Work out the finished part from the listing and answer in its coordinate system (mm). A direction names the side the tool comes from. Round coordinates to 2 decimals unless told otherwise and drop trailing zeros. Loops run counter-clockwise (first coordinate to the right, second up) from the corner with the lowest first, then second, coordinate; pieces in that order, holes last. Notation, with made-up numbers: (81.5, 39.5) -> (119.5, 39.5) arc R22 cw to (119.5, 51.5) -> close; hole circle Ø8 at (50.25, -35). An arc over 180 degrees is marked (long way). Use one line per item in the form item = value.
```python
from build123d import *

# Parameters (mm, degrees)
F0_W      = 60
F0_H      = 30
F0_W_2    = 30
F0_H_2    = 60
F1_DEPTH  = 20
F3_DEPTH  = 5
F4_W      = 5
F4_H      = 5
F5_DEPTH  = 15
F6_W      = 5
F6_H      = 5
F7_DEPTH  = 15
F8_DEPTH  = 15
F9_W      = 5
F9_H      = 5
F10_DEPTH = 15
F11_W     = 10
F11_H     = 10
F12_DEPTH = 5
F13_W     = 5
F13_H     = 2.5
F14_DEPTH = 40
F15_DEPTH = 15


# Not quite as in the source:
# - a feature names something its author has since deleted; it is built from what else it names


with BuildPart() as f1:
    # F0 (on Top) → F1 (new body)
    with BuildSketch(Plane.XY):
        with Locations((15, 30)):
            Rectangle(F0_W, F0_H)
        with Locations((-30, 30)):
            Rectangle(F0_W_2, F0_H)
        with Locations((-30, -15)):
            Rectangle(F0_W_2, F0_H_2)
    extrude(amount=F1_DEPTH)

    # F2 (on face) → F3 (cut)
    with BuildSketch(Plane(origin=(0, 0, 0), x_dir=(1, 0, 0), z_dir=(0, 0, -1))):
        Polygon((-13.218164444, -40), (45, -40), (45, -20), (-15, -20), (-20, -20), (-20, -15), (-20, 3.0019930564), (-20, 45), (-40, 45), (-37.5, -40), align=None)
    extrude(amount=-F3_DEPTH, mode=Mode.SUBTRACT)

    # F4 (on face) → F5 (join)
    with BuildSketch(Plane(origin=(0, 0, 0), x_dir=(1, 0, 0), z_dir=(0, 0, -1))):
        with Locations((32.5, -42.5)):
            Rectangle(F4_W, F4_H)
    extrude(amount=F5_DEPTH)

    # F6 (on face) → F7 (join)
    with BuildSketch(Plane(origin=(0, 0, 0), x_dir=(1, 0, 0), z_dir=(0, 0, -1))):
        with Locations((-2.5, -17.5)):
            Rectangle(F6_W, F6_H)
    extrude(amount=F7_DEPTH)

    # F6 (on face) → F8 (join)
    with BuildSketch(Plane(origin=(0, 0, 0), x_dir=(1, 0, 0), z_dir=(0, 0, -1))):
        Polygon((-20, 20), (-20, 15), (-15, 15), align=None)
    extrude(amount=F8_DEPTH)

    # F9 (on face) → F10 (join)
    with BuildSketch(Plane(origin=(0, 0, 0), x_dir=(1, 0, 0), z_dir=(0, 0, -1))):
        with Locations((-42.5, 22.5)):
            Rectangle(F9_W, F9_H)
    extrude(amount=F10_DEPTH)

    # F11 (on face) → F12 (join)
    with BuildSketch(Plane.XY.offset(20)):
        with Locations((-40, 40)):
            Rectangle(F11_W, F11_H)
    extrude(amount=F12_DEPTH)

    # F13 (on face) → F14 (cut)
    with BuildSketch(Plane.XZ.offset(-35)):
        with Locations((-40, 21.25)):
            Rectangle(F13_W, F13_H)
    extrude(amount=-F14_DEPTH, mode=Mode.SUBTRACT)

    # F4 (on face) → F15 (join)
    with BuildSketch(Plane(origin=(0, 0, 0), x_dir=(1, 0, 0), z_dir=(0, 0, -1))):
        with Locations((-42.5, -42.5)):
            Rectangle(F4_W, F4_H)
    extrude(amount=F15_DEPTH)


solid = f1.part
```
(1) Given P1, Ø1.5, axis at y = 42, z = 21.5, coming from the +X side; P2, Ø5.5, axis at x = -17.5, y = -23, coming from the -Z side; P3, Ø2.5, axis at x = -18, z = -11, coming from the +Y side, each flat-ended and moving along its own axis, determine where each tip first touches the part or whether it passes through.
Completed:
P1 = -35
P2 = 0
P3 = -15
(2) Find section A-A, the plane z = -4. Write down the section's boundary in (x, y), then the cut area to 4 significant figures.
Completed:
outline = (-45, -25) -> (-40, -25) -> (-40, -20) -> (-45, -20) -> close; (-45, 40) -> (-40, 40) -> (-40, 45) -> (-45, 45) -> close; (-20, -20) -> (-15, -15) -> (-20, -15) -> close; (-5, 15) -> (0, 15) -> (0, 20) -> (-5, 20) -> close; (30, 40) -> (35, 40) -> (35, 45) -> (30, 45) -> close
area = 112.5 mm2
(3) Find section C-C, the plane x = 13. Write down the section's boundary in (y, z), then the cut area to 3 significant figures.
Completed:
outline = (15, 0) -> (20, 0) -> (20, 5) -> (40, 5) -> (40, 0) -> (45, 0) -> (45, 20) -> (15, 20) -> close
area = 500 mm2
(4) For a pull along Z with two mould halves and no side action, classify faces 4 (the flat face through (-18, -30, 0)), 5 (the flat face through (-40, 40, 22.5)), 6 (the flat face through (-15, -15, 10)) as +Z half, -Z half, draft (parallel to the pull), parting line (faces both ways), or undercut.
Completed:
face_4 = -Z half
face_5 = undercut
face_6 = draft
(5) For faces 1 (the flat face through (15, 15, 10)), 2 (the flat face through (-18, -15, -7)), 3 (the flat face through (-16, 7, 0)), determine the directions among +Z, -Z, +X, -X, +Y, -Y from which every point of the face is accessible in a straight line to the end or side of a thin tool.
Completed:
face_1 = +Z, -Z, +X, -Y
face_2 = -Z, +X, -X, +Y
face_3 = -Z, -X, +Y
(6) Find section B-B, the plane z = 3. Write down the section's boundary in (x, y).
Completed:
outline = (-45, -45) -> (-40, -45) -> (-37.5, 40) -> (45, 40) -> (45, 45) -> (-45, 45) -> close; (-20, -45) -> (-15, -45) -> (-15, 15) -> (45, 15) -> (45, 20) -> (-20, 20) -> close
(7) Consider L1, parallel to Z at x = -24, y = 39; L2, parallel to Y at x = 11, z = 10; L3, parallel to X at y = -23.5, z = 15. Determine where each line is inside the solid, lowest interval first.
Completed:
L1 = 5 to 20
L2 = 15 to 45
L3 = -45 to -15
(8) Find section D-D, the plane y = -32.5. Write down the section's boundary in (x, z), then the cut area to 3 significant figures.
Completed:
outline = (-45, 0) -> (-39.63, 0) -> (-39.63, 5) -> (-20, 5) -> (-20, 0) -> (-15, 0) -> (-15, 20) -> (-45, 20) -> close
area = 502 mm2
